```python
from build123d import *

# Parameters (mm, degrees)
EXTRUDE1_DEPTH     = 46
SKETCH2_R          = 1.6
CUT_EXTRUDE1_DEPTH = 5000
EXTRUDE2_DEPTH     = 8
EXTRUDE3_DEPTH     = 8


with BuildPart() as part:
    # Sketch1 → Extrude1 (new body)
    with BuildSketch(Plane.XY):
        Polygon((-38.5, -40), (-18.5, -40), (-10.5, -32), (-10.5, -13), (-5.5, -8), (100.5, -8), (105.5, -13), (105.5, -32), (113.5, -40), (133.5, -40), (133.5, -32), (118.5, -32), (113.5, -27), (113.5, -9.344202483), (104.155797517, 0), (-9.155797517, 0), (-18.5, -9.344202483), (-18.5, -27), (-23.5, -32), (-38.5, -32), align=None)
    extrude(amount=-EXTRUDE1_DEPTH)

    # Sketch2 → Cut-Extrude1 (cut)
    with BuildSketch(Plane.XZ.offset(40)):
        with Locations((-30.000001952, -14.5)):
            Circle(SKETCH2_R)
        with Locations((-30.000001952, -39.5)):
            Circle(SKETCH2_R)
        with Locations((125, -14.5)):
            Circle(SKETCH2_R)
        with Locations((125, -39.5)):
            Circle(SKETCH2_R)
        with BuildLine():
            ThreePointArc((0, -16.15), (1.65, -14.5), (0, -12.85))
            ThreePointArc((0, -12.85), (-1.65, -14.5), (0, -16.15))
        make_face()
        with BuildLine():
            ThreePointArc((0, -41.15), (1.65, -39.5), (0, -37.85))
            ThreePointArc((0, -37.85), (-1.65, -39.5), (0, -41.15))
        make_face()
        with BuildLine():
            ThreePointArc((95, -16.15), (96.65, -14.5), (95, -12.85))
            ThreePointArc((95, -12.85), (93.35, -14.5), (95, -16.15))
        make_face()
        with BuildLine():
            ThreePointArc((95, -41.15), (96.65, -39.5), (95, -37.85))
            ThreePointArc((95, -37.85), (93.35, -39.5), (95, -41.15))
        make_face()
    extrude(amount=-CUT_EXTRUDE1_DEPTH, mode=Mode.SUBTRACT)

    # Sketch3 → Extrude2 (cut)
    with BuildSketch(Plane.XY):
        Polygon((-38.5, -32), (-38.5, -40), (-18.5, -40), (-10.5, -32), (-10.5, -13), (-5.5, -8), (100.5, -8), (105.5, -13), (105.5, -32), (113.5, -40), (133.5, -40), (133.5, -32), (118.5, -32), (113.5, -27), (113.5, -9.344202483), (104.155797517, 0), (-9.155797517, 0), (-18.5, -9.344202483), (-18.5, -27), (-23.5, -32), align=None)
    extrude(amount=-EXTRUDE2_DEPTH, mode=Mode.SUBTRACT)

    # Sketch4 → Extrude3 (cut)
    with BuildSketch(Plane(origin=(0, 0, 0), x_dir=(1, 0, 0), z_dir=(0, 1, 0))):
        Polygon((9.5, 46), (17.5, 38), (77.5, 38), (85.5, 46), align=None)
        Polygon((85.5, 8), (9.5, 8), (17.5, 16), (77.5, 16), align=None)
    extrude(amount=-EXTRUDE3_DEPTH, mode=Mode.SUBTRACT)


solid = part.part
```
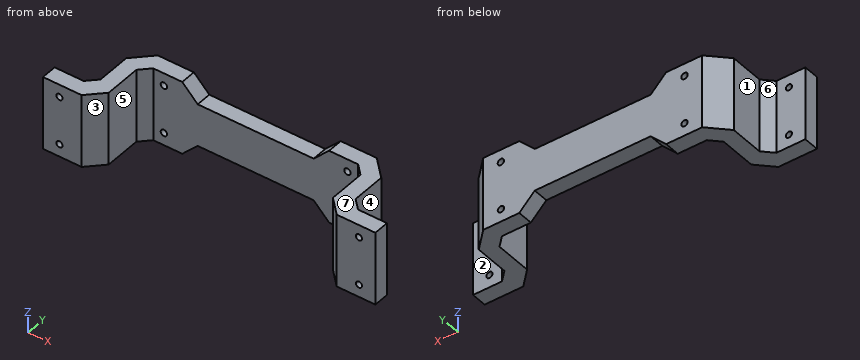
Build history of the part. All positions in model axes, mm. Face numbers are marked on the shaded views. A direction names the side the tool comes from. Round coordinates to 2 decimals unless told otherwise and drop trailing zeros. Loops run counter-clockwise (first coordinate to the right, second up) from the corner with the lowest first, then second, coordinate; pieces in that order, holes last. Notation, with made-up numbers: M 64.5,32.5 L 91.5,32.5 A19 ccw 91.5,59.5 Z; hole C 53,37 d10. An arc over 180 degrees is marked long. Answer as CSV lines item,"result".
1. Cut at D-D on x = 0. Write the cut outline in (y, z), then the cut area to 3 significant figures.
Resolved:
outline,"M -8,-46 L 0,-46 L 0,-41.15 L -8,-41.15 Z; M -8,-37.85 L 0,-37.85 L 0,-16.15 L -8,-16.15 Z; M -8,-12.85 L 0,-12.85 L 0,-8 L -8,-8 Z"
area,"251 mm²"
2. Cut at A-A on y = -35. Write the cut outline in (x, z), then the cut area to 3 significant figures.
Resolved:
outline,"M -38.5,-46 L -13.5,-46 L -13.5,-8 L -38.5,-8 Z; M 108.5,-46 L 133.5,-46 L 133.5,-8 L 108.5,-8 Z; hole C -30,-39.5 d3.2; hole C -30,-14.5 d3.2; hole C 125,-39.5 d3.2; hole C 125,-14.5 d3.2"
area,"1,870 mm²"
3. Flat gauge pins, fed straight in: P1, Ø4, axis at x = 58, y = -3.5, coming from the +Z side; P2, Ø7.5, axis at x = -32, z = -20.5, coming from the +Y side; P3, Ø11.5, axis at x = 44.5, z = -32.5, coming from the -Y side. Where does each tip first touch, or does it go through?
Resolved:
P1,"stops at z = -16"
P2,"stops at y = -32"
P3,"stops at y = -8"
4. Cut at C-C on z = -22. Write the cut outline in (x, y), then the cut area to 3 significant figures.
Resolved:
outline,"M -38.5,-40 L -18.5,-40 L -10.5,-32 L -10.5,-13 L -5.5,-8 L 100.5,-8 L 105.5,-13 L 105.5,-32 L 113.5,-40 L 133.5,-40 L 133.5,-32 L 118.5,-32 L 113.5,-27 L 113.5,-9.34 L 104.16,0 L -9.16,0 L -18.5,-9.34 L -18.5,-27 L -23.5,-32 L -38.5,-32 Z"
area,"1,790 mm²"
5. Cut at B-B on x = 125. Write the cut outline in (y, z), then the cut area to 3 significant figures.
Resolved:
outline,"M -40,-46 L -32,-46 L -32,-41.1 L -40,-41.1 Z; M -40,-37.9 L -32,-37.9 L -32,-16.1 L -40,-16.1 Z; M -40,-12.9 L -32,-12.9 L -32,-8 L -40,-8 Z"
area,"253 mm²"
6. Wall check: probe 1 along Z at (x, y) = (125, -36.5); probe 2 along X at (y, z) = (-1.5, -14.5); probe 3 along Y at (x, z) = (122, -15.5). Give the ranges that are in metal, low to high. Write a range as [from, to].
Resolved:
probe 1,"z = [-46, -41.1], [-37.9, -16.1], [-12.9, -8]"
probe 2,"x = [-10.66, -1.65], [1.65, 16], [79, 93.35], [96.65, 105.66]"
probe 3,"y = [-40, -32]"
7. 3-axis set-ups, long thin cutter, end or side, ignore diameter. For the marked faces 1, 2 and 3: which of +Z, -Z, +X, -X, +Y, -Y reach the whole face in a straight line?
Resolved:
face 1,"+Z, -Z, -X, +Y"
face 2,"+Z, -Z, +X, +Y"
face 3,"+Z, -Z, -Y"
8. Two-plate mould, pull along X, no slides. Class the marked faces 4, 5, 6 and 7: released by +X, released by -X, zero draft, split by the parting line, or undercut.
Resolved:
face 4,"released by +X"
face 5,"undercut"
face 6,"released by -X"
face 7,"zero draft"
